Here's how the part is built. I have some questions about the finished solid (model axes, mm). Face numbers are marked on the shaded views. A direction names the side the tool comes from. Give positions to 0.01 mm unless a question says otherwise; leave off trailing zeros. Loops run counter-clockwise (first coordinate to the right, second up) from the corner with the lowest first, then second, coordinate; pieces in that order, holes last. Notation, with made-up numbers: (44.25, 23.25) - (92.25, 23.25) arc R25 ccw to (92.25, 59.25) - close; hole circle Ø3 at (11.5, -24.5). An arc over 180 degrees is marked (long way). Use one line per item in the form item = value.
from build123d import *

# Parameters (mm, degrees)
F1_DEPTH = 5
F0_R     = 1.75
F2_DEPTH = 2
F3_R     = 2
F4_R     = 1


with BuildPart() as f1:
    # F0 (on Top) → F1 (new body)
    with BuildSketch(Plane.XY):
        with BuildLine():
            Line((-57.497826, 24.5), (-68.5, 24.5))
            Line((-68.5, 24.5), (-62.5, 0))
            ThreePointArc((-62.5, 0), (-61.236689, 12.502717), (-57.497826, 24.5))
        make_face()
    extrude(amount=F1_DEPTH)

    # F0 (on Top) → F2 (join)
    with BuildSketch(Plane.XY):
        with BuildLine():
            Line((-68.5, 24.5), (-82.5, 24.5))
            Line((-82.5, 24.5), (-82.5, -24.5))
            Line((-82.5, -24.5), (-57.497826, -24.5))
            ThreePointArc((-57.497826, -24.5), (-61.236689, -12.502717), (-62.5, 0))
            Line((-62.5, 0), (-68.5, 24.5))
        make_face()
        with Locations((-77.5, 0)):
            Circle(F0_R, mode=Mode.SUBTRACT)
    extrude(amount=F2_DEPTH)

    # F3
    f3_edges = [f1.edges().sort_by_distance(p)[0] for p in [
        (-82.5, -24.5, 1),
        (-82.5, 24.5, 1),
    ]]
    fillet(f3_edges, radius=F3_R)

    # F4
    f4_edges = [f1.edges().sort_by_distance(p)[0] for p in [
        (-65.5, 12.25, 5),
    ]]
    fillet(f4_edges, radius=F4_R)


solid = f1.part
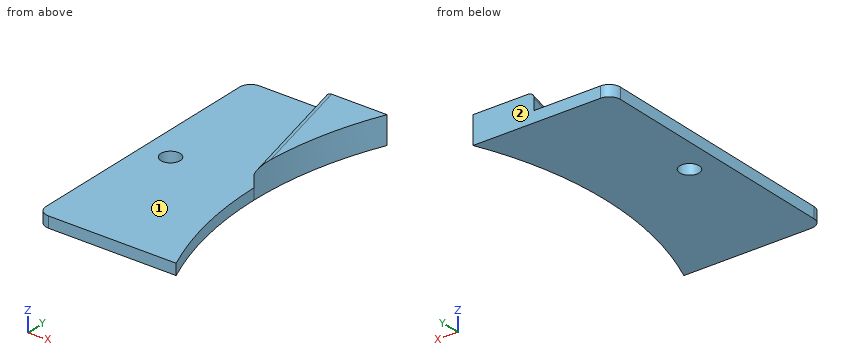
(1) If we section it at B-B (z = 1.5): List the corners of the cut face in (x, y) for me, plus the area to 3 significant figures.
Geometry says:
outline = (-82.5, -22.5) arc R2 ccw to (-80.5, -24.5) - (-57.5, -24.5) arc R62.5 cw to (-62.5, 0) arc R62.5 cw to (-57.5, 24.5) - (-80.5, 24.5) arc R2 ccw to (-82.5, 22.5) - close; hole circle Ø3.5 at (-77.5, 0)
area = 1,050 mm²
(2) If we section it at A-A (x = -77.5): List the corners of the cut face in (y, z) for me.
Geometry says:
outline = (-24.5, 0) - (-1.75, 0) - (-1.75, 2) - (-24.5, 2) - close; (1.75, 0) - (24.5, 0) - (24.5, 2) - (1.75, 2) - close
(3) If I drill on probe 1 along Y at (x, z) = (-77.5, 1); probe 2 along Z at (x, y) = (-74.25, 22); probe 3 along X at (y, z) = (20.5, 1.25), over which ranges is the centre line in solid material (lowest first)?
Geometry says:
probe_1 = -24.5 to -1.75, 1.75 to 24.5
probe_2 = 0 to 2
probe_3 = -82.5 to -59.04
(4) If we section it at D-D (y = -8.5): List the corners of the cut face in (x, z) for me, plus the area to 3 significant figures.
Geometry says:
outline = (-82.5, 0) - (-61.92, 0) - (-61.92, 2) - (-82.5, 2) - close
area = 41.2 mm²
(5) If we section it at C-C (x = -61.5): List the corners of the cut face in (y, z) for me.
Geometry says:
outline = (-24.5, 0) - (-11.14, 0) - (-11.14, 2) - (-24.5, 2) - close; (11.14, 0) - (24.5, 0) - (24.5, 5) - (11.14, 5) - close
(6) For P1, Ø3, axis at x = -65, y = 7.5, coming from the +Z side; P2, Ø2, axis at y = 6, z = 4, coming from the +X side; P3, Ø1.5, axis at y = 12.5, z = 2, coming from the +X side, each with a flat end and sliding along its axis, tell me the tip position at first contact or that it passes through.
Geometry says:
P1 = 4.99
P2 = -62.11
P3 = -61.08
(7) For the marked faces 1 and 2, which set-ups out of +Z, -Z, +X, -X, +Y, -Y let a thin tool reach every point of the face, with its end or its side?
Geometry says:
face_1 = +Z, -X, -Y
face_2 = +Z, -Z, +X, -X, +Y
